The listing builds one solid part. Answer for the finished solid, in the listing's coordinates (mm). A direction names the side the tool comes from. Give positions to 0.01 mm unless a question says otherwise; leave off trailing zeros. Order: outer loops, then holes, each group sorted by start corner. A loop starts at its lowest first (then second) coordinate and runs counter-clockwise, first axis right, second up. Notation, with made-up numbers: (87.5, 8) - (110.5, 8) arc R12 ccw to (110.5, 27) - close; hole circle Ø1 at (5, -4.5). An arc over 180 degrees is marked (long way). Write each question's results on one line, items separated by ' | '. Start each with the question number.
1. Section B-B (z = 5.75) is taken. Give the vertices of the cut face in (x, y).
2. Determine the mould class of faces 1 (the face through (-0.348, -0.014, 21.227)), 2 (the face through (0.041, -2.211, 14.703)), 3 (the face through (-1.349, -2.397, 7.353)) for opening direction X: released by +X, released by -X, zero draft, split by the parting line, or undercut.
3. Find the intervals of material crossed by L1, parallel to Z at x = 0, y = -1.25; L2, parallel to X at y = -0.75, z = 5; L3, parallel to Y at x = 0.75, z = 14, in increasing order.
4. Section C-C (y = 2.25) is taken. Give the vertices of the cut face in (x, z).
5. Section A-A (z = 18.5) is taken. Give the vertices of the cut face in (x, y), and give its area (3 significant figures).
6. Flat-ended cylindrical pins translate along their axes: pin 1 (4 mm diameter, centred on x = -3, z = 16, fed in from -Y); pin 2 (2.5 mm diameter, centred on x = -2, z = 20, fed in from +Y). Find the tip coordinate at first contact, or state that the pin passes through.
7. Which of the six approach directions +Z, -Z, +X, -X, +Y, -Y give full straight-line access (tool end or side, diameter ignored) to faces 4 (the face through (1.349, 2.397, 7.358)), 5 (the face through (0.1, -1.579, 21.4)), 6 (the face through (-1.401, 2.366, 7.358)), 7 (the face through (1.401, -2.366, 7.357))?
Autodesk Inventor part; units mm, degrees
ref_plane "Plano de trabajo4" through (-2.7452, -1.596, 0) normal (0, 0, -1) x (-1, 0, 0)
ref_plane "Plano de trabajo5" through (0, -3.175, 0) normal (0, 1, 0) x (-1, 0, 0)
ref_plane "Barreno" through (0, 0, 0) normal (0, -1, 0) x (1, 0, 0)
sketch "Boceto1" plane through (0, 0, 0) normal (0, 0, 1) x (1, 0, 0)
  line L0 (2.7452, 1.596) -> (2.7548, -1.5794)
  line L1 (2.7548, -1.5794) -> (0.0096, -3.1754)
  line L2 (0.0096, -3.1754) -> (-2.7452, -1.596)
  line L3 (-2.7452, -1.596) -> (-2.7548, 1.5794)
  line L4 (-2.7548, 1.5794) -> (-0.0096, 3.1754)
  line L5 (-0.0096, 3.1754) -> (2.7452, 1.596)
  point P0 (0, 0)
  point P1 (0, 0)
  dimension "d0" = 5.5
  dimension "d20" = 6.3508
extrude "Extrusión1" add sketch "Boceto1" along normal blind 15
ref_plane "Plano de trabajo4" through (-2.7452, -1.596, 0) normal (0, 0, -1) x (-1, 0, 0)
sketch "Boceto2" plane through (-2.7452, -1.596, 0) normal (0, 0, -1) x (-1, 0, 0)
  line L0 (-2.7548, -1.5794) -> (1.0358, -1.5794)
  line L1 (1.0358, -1.5794) -> (-2.7548, -1.5794)
  line L2 (-5.6299, -1.5794) -> (-2.7548, -1.5794)
  point P0 (-2.7452, 1.596)
  dimension "d5" = 3.1754
ref_plane "Plano de trabajo5" through (0, -3.175, 0) normal (0, 1, 0) x (-1, 0, 0)
sketch "Boceto3" plane through (0, -3.175, 0) normal (0, 1, 0) x (-1, 0, 0)
  line L0 (-0.0096, 15) -> (-2.7548, 15)
  line L1 (2.6199, 14) -> (-2.7548, 14) construction
  line L2 (-0.0096, 0) -> (-0.0096, 15)
  line L3 (-0.0096, 14) -> (-0.0096, 18.5)
  circle A0 centre (-0.0096, 18.5) radius 4.25
  circle A1 centre (-0.0096, 18.5) radius 2.75
  point P0 (0, 0)
  dimension "d7" = 1
  dimension "d8" = 4.5
  dimension "d9" = 8.5
  dimension "d14" = 5.5
sketch "Boceto4" plane through (-2.7452, -1.596, 0) normal (0, 0, -1) x (-1, 0, 0)
  point P0 (-2.7452, 1.596)
  point P1 (-2.7356, 4.7714)
  point P2 (-2.7548, -1.579)
  dimension "d10" = 6.3504
extrude "Extrusión2" add sketch "Boceto3" along normal blind 6.35 contours L2 A0 L0 | L0 A0 L2 | A1
ref_plane "Barreno" through (0, 0, 0) normal (0, -1, 0) x (1, 0, 0)
sketch "Boceto6" plane through (0, 0, 0) normal (0, -1, 0) x (1, 0, 0)
  arc A0 (0.0103, 14.25) -> (0.0089, 14.25) centre (0.0096, 18.5) ccw
  circle A1 centre (0.0096, 18.5) radius 2.75
  point P0 (0, 0)
  dimension "d13" = 4.25
extrude "Extrusión3" cut sketch "Boceto6" along normal mid plane 10 contours A1
ref_plane "Plano de trabajo8" through (5, 0, 0) normal (1, 0, 0) x (0, 1, 0)
sketch "Boceto8" plane through (5, 0, 0) normal (1, 0, 0) x (0, 1, 0)
  line L0 (-3.175, 15.75) -> (-3.175, 21.25)
  line L1 (-3.1754, 14.25) -> (-1.5794, 15)
  line L2 (-1.5794, 15) -> (-1.5794, 22.75)
  line L3 (-1.5794, 22.75) -> (-3.175, 22.75)
  line L4 (3.175, 14.25) -> (1.596, 15)
  line L5 (1.596, 15) -> (1.596, 22.75)
  line L6 (1.596, 22.75) -> (3.175, 22.75)
  ellipse E0 centre (3.1866, 18.5) end of major axis (3.1866, 14.25) minor radius 2.4709 (1.7849, 15) -> (3.175, 14.25) ccw
  line L7 (-3.175, 22.75) -> (-6.1952, 22.75)
  line L8 (-6.1952, 22.75) -> (-6.1952, 14.0055)
  line L9 (-6.1952, 14.0055) -> (-3.1754, 14.25)
  line L10 (3.175, 14.25) -> (7.2865, 13.4418)
  line L11 (7.2865, 13.4418) -> (6.5328, 22.75)
  line L12 (6.5328, 22.75) -> (3.175, 22.75)
  point P0 (0, 0)
  point P1 (-1.5794, 15)
extrude "Extrusión4" cut sketch "Boceto8" against normal blind 10 contours L9 L8 L7 L3 L2 L1 | L4 L5 L6 L12 L11 L10
fillet "Empalme1" radius 2 1 edges at (-2.75, 0, 15)
fillet "Empalme2" radius 2 1 edges at (2.75, 0.0083, 15)
properties part number "Cabezal" material "Plástico ABS"
Reported:
1) outline: (-2.75, -1.6) - (0.01, -3.18) - (2.75, -1.58) - (2.75, 1.6) - (-0.01, 3.18) - (-2.75, 1.58) - close
2) face 1: undercut | face 2: zero draft | face 3: released by -X
3) L1: 0 to 15.75, 21.25 to 22.75 | L2: -2.75 to 2.75 | L3: -2.74 to 2.74
4) outline: (-1.87, 14.69) arc R4.25 ccw to (-1.6, 14.57) - (-1.6, 0) - (1.6, 0) - (1.6, 14.56) arc R4.25 ccw to (1.89, 14.69) - close
5) outline: (-4.24, -1.58) - (-2.74, -1.58) - (-2.74, 1.6) - (-4.24, 1.6) - close; (2.76, -1.58) - (4.26, -1.58) - (4.26, 1.6) - (2.76, 1.6) - close | area: 9.53 mm²
6) pin 1: y = -2.5 | pin 2: y = 1.6
7) face 4: -Z, +X, +Y | face 5: +Z, +X, -X, -Y | face 6: -Z, -X, +Y | face 7: -Z, +X, -Y
